Verification items for the finished model (mm, model axes). Face numbers are marked on the shaded views. A direction names the side the tool comes from. Coordinates: 2 decimals unless noted, no trailing zeros. Loops run counter-clockwise (first coordinate to the right, second up) from the corner with the lowest first, then second, coordinate; pieces in that order, holes last. Notation, with made-up numbers: (86, 75.5) - (139, 75.5) arc R15 ccw to (139, 91.5) - close; hole circle Ø1 at (-36.75, 31). An arc over 180 degrees is marked (long way). One line per item, written item: value. Start each with the question number.
(1) Thickness scan on probe 1 along X at (y, z) = (125, -5.25); probe 2 along Y at (x, z) = (-8.5, 7.5); probe 3 along Y at (x, z) = (0, -7.6). Record the ranges inside material, lowest first. Write a range as [from, to].
(2) Set-up check for the marked faces 5, 6 and 7: record each of +Z, -Z, +X, -X, +Y, -Y from which the full face is reachable in a straight line by a thin tool's end or side.
(3) Section check A-A (y = 125). Record the boundary of the cut face in (x, z), plus the area to 3 significant figures.
(4) Gauge pin test, flat ends, axial feed: P1, Ø1.6, axis at y = 87.5, z = 9, coming from the -X side; P2, Ø1.5, axis at y = 63.5, z = 1, coming from the +X side; P3, Ø3, axis at x = -19, z = 2.5, coming from the +Y side; P4, Ø5, axis at x = 2.5, z = 6, coming from the -Y side. Record the tip position at first contact, or that the pin passes through.
(5) Section check B-B (x = 0). Record the boundary of the cut face in (y, z).
(6) Draft check along Y on the marked faces 1, 2, 3 and 4. Enter one of: +Y half, -Y half, draft (parallel to the pull), parting line (faces both ways), or undercut.
```python
from build123d import *

# Parameters (mm, degrees)
SKETCH1_R                         = 6.5
BOSS_EXTRUDE1_DEPTH               = 10
SKETCH2_R                         = 14
CUT_EXTRUDE1_DEPTH                = 14
CHAMFER1_SIZE                     = 4
CHAMFER2_SIZE                     = 1
FILLET2_R                         = 5
CUT_EXTRUDE2_DEPTH                = 4
FILLET3_R                         = 2
FILLET3_OF_MIRROR1_R              = 2
M10X1_25_TAPPED_HOLE1_D           = 8.8
M10X1_25_TAPPED_HOLE1_DEPTH       = 20
M10X1_25_TAPPED_HOLE1_CSINK_D     = 10.05
M10X1_25_TAPPED_HOLE1_CSINK_ANGLE = 90
M10X1_25_TAPPED_HOLE1_TIP         = 2.643786724


with BuildPart() as part:
    # Sketch1 → Boss-Extrude1 (new, symmetric)
    with BuildSketch(Plane.XY):
        with BuildLine():
            Line((-47.170361299, 15), (-47.170361299, 0))
            Line((-47.170361299, 0), (47.170361299, 0))
            Line((47.170361299, 0), (47.170361299, 15))
            Line((47.170361299, 15), (30, 80))
            Line((30, 80), (30, 137))
            Line((30, 137), (16, 137))
            ThreePointArc((16, 137), (0, 145), (-16, 137))
            Line((-16, 137), (-30, 137))
            Line((-30, 137), (-30, 80))
            Line((-30, 80), (-47.170361299, 15))
        make_face()
        with Locations((0, 125)):
            Circle(SKETCH1_R, mode=Mode.SUBTRACT)
    extrude(amount=BOSS_EXTRUDE1_DEPTH, both=True)

    # Sketch2 → Cut-Extrude1 (cut)
    with BuildSketch(Plane.XY.offset(10)):
        with Locations((0, 125)):
            Circle(SKETCH2_R)
    extrude(amount=-CUT_EXTRUDE1_DEPTH, mode=Mode.SUBTRACT)

    # Chamfer1
    chamfer1_edges = [part.edges().sort_by_distance(p)[0] for p in [
        (30, 137, 0),
        (-30, 137, 0),
    ]]
    chamfer(chamfer1_edges, length=CHAMFER1_SIZE)

    # Chamfer2
    chamfer2_edges = [part.edges().sort_by_distance(p)[0] for p in [
        (-14, 125, 10),
    ]]
    chamfer(chamfer2_edges, length=CHAMFER2_SIZE)

    # Fillet2
    fillet2_edges = [part.edges().sort_by_distance(p)[0] for p in [
        (-16, 137, 0),
        (16, 137, 0),
    ]]
    fillet(fillet2_edges, radius=FILLET2_R)

    # Sketch3 → Cut-Extrude2 (cut)
    with BuildSketch(Plane.XY.offset(10)):
        with BuildLine():
            Line((-10, 100), (10, 100))
            ThreePointArc((10, 100), (15.656854249, 97.656854249), (18, 92))
            Line((18, 92), (18, 78.441768634))
            Line((18, 78.441768634), (30.784939674, 30.043190159))
            ThreePointArc((30.784939674, 30.043190159), (29.388451789, 23.118684669), (23.050253256, 20))
            Line((23.050253256, 20), (-23.050253256, 20))
            ThreePointArc((-23.050253256, 20), (-29.388451789, 23.118684669), (-30.784939674, 30.043190159))
            Line((-30.784939674, 30.043190159), (-18, 78.441768634))
            Line((-18, 78.441768634), (-18, 92))
            ThreePointArc((-18, 92), (-15.656854249, 97.656854249), (-10, 100))
        make_face()
    cut_extrude2 = extrude(amount=-CUT_EXTRUDE2_DEPTH, mode=Mode.SUBTRACT)

    # Fillet3
    fillet3_edges = [part.edges().sort_by_distance(p)[0] for p in [
        (-29.388451789, 23.118684669, 6),
        (-24.392469837, 54.242479397, 6),
        (-18, 85.220884317, 6),
        (-15.656854249, 97.656854249, 6),
        (0, 100, 6),
        (15.656854249, 97.656854249, 6),
        (18, 85.220884317, 6),
        (24.392469837, 54.242479397, 6),
        (29.388451789, 23.118684669, 6),
        (0, 20, 6),
    ]]
    fillet(fillet3_edges, radius=FILLET3_R)

    # Mirror1: Cut-Extrude2 across plane
    add(cut_extrude2.mirror(Plane.XY), mode=Mode.SUBTRACT)

    # Fillet3 of Mirror1
    fillet3_of_mirror1_edges = [part.edges().sort_by_distance(p)[0] for p in [
        (-29.388451789, 23.118684669, -6),
        (-24.392469837, 54.242479397, -6),
        (-18, 85.220884317, -6),
        (-15.656854249, 97.656854249, -6),
        (0, 100, -6),
        (15.656854249, 97.656854249, -6),
        (18, 85.220884317, -6),
        (24.392469837, 54.242479397, -6),
        (29.388451789, 23.118684669, -6),
        (0, 20, -6),
    ]]
    fillet(fillet3_of_mirror1_edges, radius=FILLET3_OF_MIRROR1_R)

    # M10x1.25 Tapped Hole1
    with Locations(Plane(origin=(0, 0, 0), x_dir=(-1, 0, 0), z_dir=(0, -1, 0))):
        with Locations((-31.170361299, 0), (28.829638701, 0)):
            CounterSinkHole(M10X1_25_TAPPED_HOLE1_D / 2, M10X1_25_TAPPED_HOLE1_CSINK_D / 2, depth=M10X1_25_TAPPED_HOLE1_DEPTH, counter_sink_angle=M10X1_25_TAPPED_HOLE1_CSINK_ANGLE)
            with Locations((0, 0, -(M10X1_25_TAPPED_HOLE1_DEPTH + M10X1_25_TAPPED_HOLE1_TIP / 2))):  # 118° drill point
                Cone(0, M10X1_25_TAPPED_HOLE1_D / 2, M10X1_25_TAPPED_HOLE1_TIP, mode=Mode.SUBTRACT)


solid = part.part
```
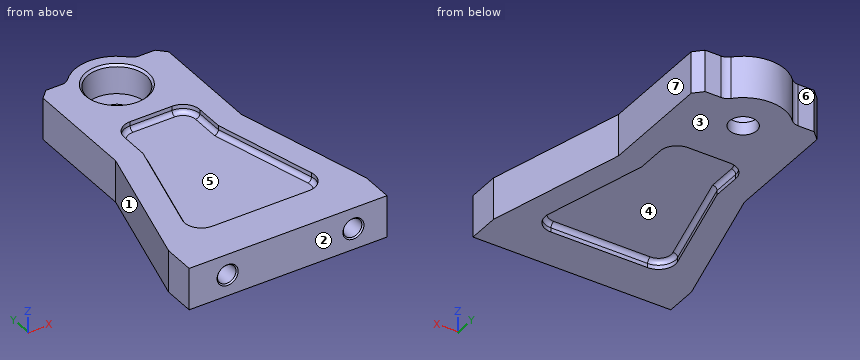
Responses:
1. probe 1: x = [-30, -6.5], [6.5, 30]
1. probe 2: y = [0, 20.06], [99.94, 113.88], [136.12, 143.1]
1. probe 3: y = [0, 20.04], [99.96, 118.5], [131.5, 145]
2. face 5: +Z
2. face 6: +Z, -Z, -X, +Y
2. face 7: +Z, -Z, +X, +Y
3. outline: (-30, -10) - (-6.5, -10) - (-6.5, -4) - (-14, -4) - (-14, 9) - (-15, 10) - (-30, 10) - close; (6.5, -10) - (30, -10) - (30, 10) - (15, 10) - (14, 9) - (14, -4) - (6.5, -4) - close
3. area: 729 mm²
4. P1: stops at x = -30
4. P2: stops at x = 34.56
4. P3: stops at y = 137.07
4. P4: stops at y = 0
5. outline: (0, -10) - (20, -10) - (20, -8) arc R2 cw to (22, -6) - (98, -6) arc R2 cw to (100, -8) - (100, -10) - (118.5, -10) - (118.5, -4) - (111, -4) - (111, 9) - (110, 10) - (100, 10) - (100, 8) arc R2 cw to (98, 6) - (22, 6) arc R2 cw to (20, 8) - (20, 10) - (0, 10) - close; (131.5, -10) - (145, -10) - (145, 10) - (140, 10) - (139, 9) - (139, -4) - (131.5, -4) - close
6. face 1: +Y half
6. face 2: -Y half
6. face 3: draft
6. face 4: undercut
